Here's the drawing with two shaded views (mm, measured from the low corner). I have some questions. A direction names the side the tool comes from. Coordinates: 2 decimals unless noted, no trailing zeros. Order: outer loops, then holes, each group sorted by start corner. A loop starts at its lowest first (then second) coordinate and runs counter-clockwise, first axis right, second up. Notation, with made-up numbers: (-15, 60.25) - (12, 60.25) arc R13 ccw to (12, 76.25) - close; hole circle Ø4 at (50.25, 52). An arc over 180 degrees is marked (long way). Answer as a JSON object with one key per item and string values. Group by question number.
(1) Please list where these lines run through material, in increasing order: probe 1 along Z at (x, y) = (4.25, 3.25); probe 2 along Z at (x, y) = (8.25, 7); probe 3 along X at (y, z) = (9.5, 1.7).
(2) Will these pins go through, and if not, where does the flat tip stop? P1, Ø1.5, axis at y = 3, z = 0.5, coming from the -X side; P2, Ø1, axis at x = 17, z = 3, coming from the +Y side; P3, Ø1.5, axis at x = 17, y = 19, coming from the -Z side; P4, Ø2, axis at y = 14.5, z = 3, coming from the +X side.
(3) Imagine slicing it at D-D, the plane y = 18. Write out the boundary of the cut face in (x, z), and give its area (3 significant figures).
(4) Imagine slicing it at C-C, the plane z = 2.95. Write out the boundary of the cut face in (x, y), and give its area (3 significant figures).
(5) Imagine slicing it at A-A, the plane y = 11. Write out the boundary of the cut face in (x, z), and give its area (3 significant figures).
(6) Which directions (+Z, -Z, +X, -X, +Y, -Y) give clear straight access to the entire face, cutting with the end or side of a thin tool? Please do the marked faces 1 and 2.
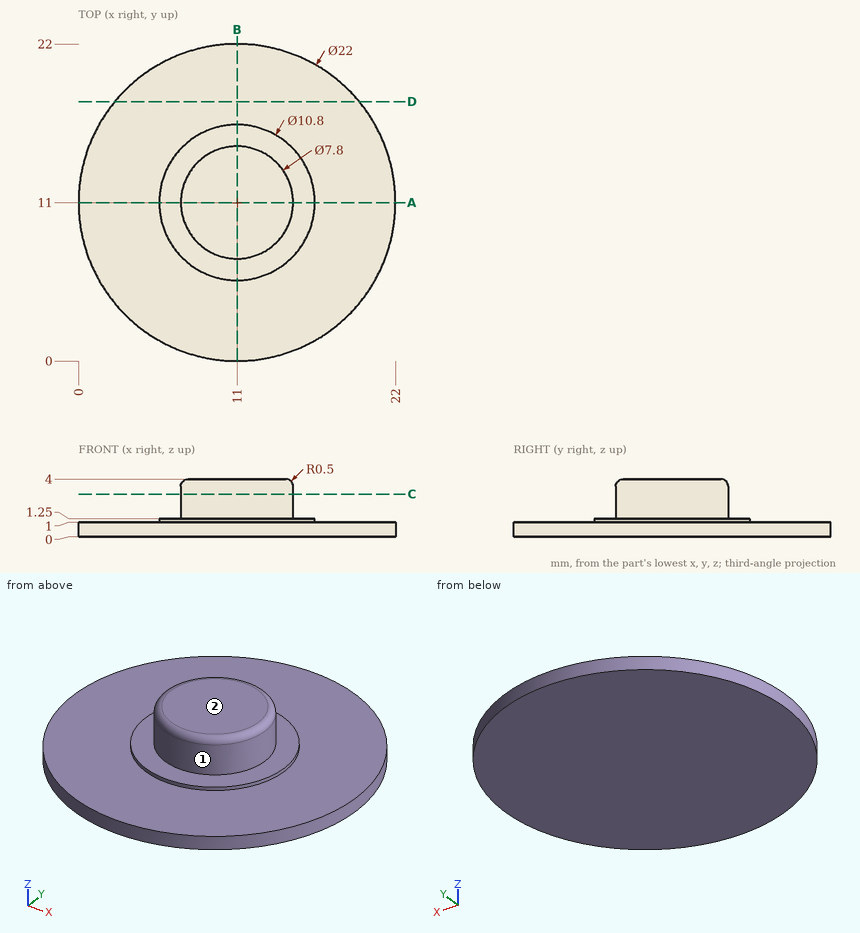
Result set:
{
 "1": {"probe 1": "z = 0 to 1", "probe 2": "z = 0 to 1.25", "probe 3": "x = 7.4 to 14.6"},
 "2": {"P1": "stops at x = 2.73", "P2": "passes through", "P3": "stops at z = 0", "P4": "stops at x = 13.99"},
 "3": {"outline": "(2.51, 0) - (19.49, 0) - (19.49, 1) - (2.51, 1) - close", "area": "17.0 mm^2"},
 "4": {"outline": "circle Ø7.8 at (11, 11)", "area": "47.8 mm^2"},
 "5": {"outline": "(0, 0) - (22, 0) - (22, 1) - (16.4, 1) - (16.4, 1.25) - (14.9, 1.25) - (14.9, 3.5) arc R0.5 ccw to (14.4, 4) - (7.6, 4) arc R0.5 ccw to (7.1, 3.5) - (7.1, 1.25) - (5.6, 1.25) - (5.6, 1) - (0, 1) - close", "area": "46.0 mm^2"},
 "6": {"face 1": "+Z", "face 2": "+Z, +X, -X, +Y, -Y"}
}
